Work out the finished part from the listing and answer in its coordinate system (mm). Face numbers are marked on the shaded views. A direction names the side the tool comes from. Coordinates: 2 decimals unless noted, no trailing zeros. Write each loop counter-clockwise with the first axis right and the second up, starting at its lowest first coordinate (ties: lowest second). Pieces come first, ordered by that corner, then holes. Notation, with made-up numbers: (-4.75, 19.25) - (54.25, 19.25) arc R15 ccw to (54.25, 36.25) - close; hole circle Ø3 at (79, 42). An arc over 180 degrees is marked (long way). Use a Markdown table: item, result. Add a question column.
(1) For a pull along Z with two mould halves and no side action, classify the marked faces 1, 2, 3 and 4 as released by +Z, released by -Z, zero draft, split by the parting line, or undercut.
(2) The part is cut by section A-A, the plane z = -13.5. Give the vertices of the cut face in (x, y).
(3) Find the intervals of material crossed by line 1 (Y direction, x = -0.2, z = -13.5); line 2 (Z direction, x = 2.25, y = -1); line 3 (Z direction, x = 0.25, y = -6), in increasing order. Write a range as from..to.
(4) The part is cut by section D-D, the plane z = -9. Give the vertices of the cut face in (x, y).
(5) Given pin 1 Ø1.8 at (x, y) = (-5, 1.5) entering from -Z; pin 2 Ø2 at (x, y) = (7, -7.5) entering from -Z; pin 3 Ø8 at (x, z) = (2, -9) entering from +Y, each flat-ended and moving along its own axis, determine where each tip first touches the part or whether it passes through.
(6) The part is cut by section B-B, the plane x = 0. Give the vertices of the cut face in (y, z).
(7) A tool of negligible diameter and unlimited length cuts with its end or side. For the marked faces 5, 6, 7 and 8, from which of +Z, -Z, +X, -X, +Y, -Y can it reach the whole face along a straight path? Write none if from no direction.
(8) The part is cut by section C-C, the plane y = 0. Give the vertices of the cut face in (x, z), then the cut area to 3 significant figures.
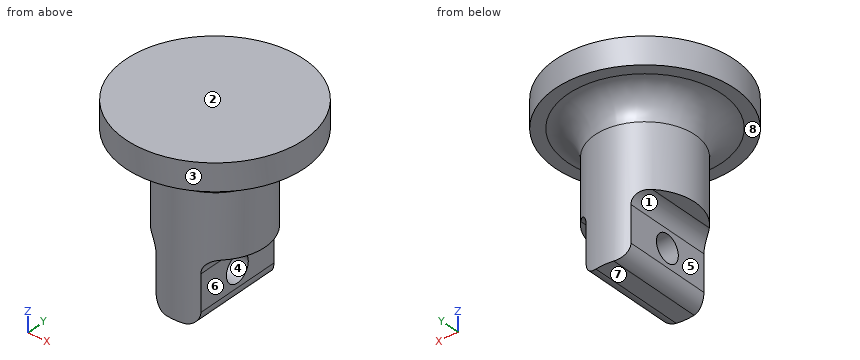
from build123d import *
from OCP.BRepFilletAPI import BRepFilletAPI_MakeFillet

# Parameters (mm, degrees)
SKETCH1_R           = 10
BOSS_EXTRUDE1_DEPTH = 3
SKETCH2_R           = 5.6
BOSS_EXTRUDE2_DEPTH = 17
CUT_EXTRUDE1_DEPTH  = 7
CUT_EXTRUDE2_REACH  = 25.351
SKETCH4_R           = 1.5
FILLET1_R1          = 3
FILLET1_R2          = 1.5


with BuildPart() as part:
    # Sketch1 → Boss-Extrude1 (new body)
    with BuildSketch(Plane.XY):
        Circle(SKETCH1_R)
    extrude(amount=BOSS_EXTRUDE1_DEPTH)

    # Sketch2 → Boss-Extrude2 (add)
    with BuildSketch(Plane(origin=(0, 0, 0), x_dir=(-1, 0, 0), z_dir=(0, 0, -1))):
        with Locations(Location((0, 0, 0), (0, 0, 180))):
            Circle(SKETCH2_R)
    extrude(amount=BOSS_EXTRUDE2_DEPTH)

    # Sketch3 → Cut-Extrude1 (cut)
    with BuildSketch(Plane(origin=(0, 0, -17), x_dir=(-1, 0, 0), z_dir=(0, 0, -1))):
        with BuildLine():
            Line((2.5, 0), (2.5, 6.663171691))
            ThreePointArc((2.5, 6.663171691), (8.066213365, -0.537352556), (2.5, -7.737876802))
            Line((2.5, -7.737876802), (2.5, 0))
        make_face()
        with BuildLine():
            Line((-2.5, 0), (-2.5, 6.663171691))
            ThreePointArc((-2.5, 6.663171691), (-7.668145551, -0.537352556), (-2.5, -7.737876802))
            Line((-2.5, -7.737876802), (-2.5, 0))
        make_face()
    extrude(amount=-CUT_EXTRUDE1_DEPTH, mode=Mode.SUBTRACT)

    # Sketch4 → Cut-Extrude2 (cut, up to next)
    with BuildSketch(Plane(origin=(2.5, 0, 0), x_dir=(0, 0, -1), z_dir=(1, 0, 0)), mode=Mode.PRIVATE) as cut_extrude2_sk1:
        with Locations((13.5, 0)):
            Circle(SKETCH4_R)
    cut_extrude2_tool1 = extrude(cut_extrude2_sk1.sketch, amount=-CUT_EXTRUDE2_REACH, mode=Mode.PRIVATE) & part.part
    add(cut_extrude2_tool1.solids().sort_by_distance((2.5, 0, -13.5))[0], mode=Mode.SUBTRACT)

    # Fillet1: one fillet with a radius per group of edges: ONE call of the kernel's fillet builder (fillet() takes one radius for all edges)
    fillet1_edges_1 = [part.edges().sort_by_distance(p)[0] for p in [
        (-5.6, 0, 0),
    ]]
    fillet1_edges_2 = [part.edges().sort_by_distance(p)[0] for p in [
        (2.5, 0, -10),
        (-2.5, 0, -10),
        (2.5, 0, -17),
        (-2.5, 0, -17),
    ]]
    fillet1 = BRepFilletAPI_MakeFillet(part.part.solid().wrapped)
    for e in fillet1_edges_1:
        fillet1.Add(FILLET1_R1, e.wrapped)
    for e in fillet1_edges_2:
        fillet1.Add(FILLET1_R2, e.wrapped)
    add(Compound.cast(fillet1.Shape()), mode=Mode.REPLACE)


solid = part.part
Model answer:
| question | item | result |
|---|---|---|
| 1 | face 1 | released by -Z |
| 1 | face 2 | released by +Z |
| 1 | face 3 | zero draft |
| 1 | face 4 | undercut |
| 2 | outline | (-2.5, -5.01) arc R5.6 ccw to (2.5, -5.01) - (2.5, -1.5) - (-2.5, -1.5) - close; (-2.5, 1.5) - (2.5, 1.5) - (2.5, 5.01) arc R5.6 ccw to (-2.5, 5.01) - close |
| 3 | line 1 | -5.6..-1.5, 1.5..5.6 |
| 3 | line 2 | -16.33..-14.62, -12.38..3 |
| 3 | line 3 | -1.49..3 |
| 4 | outline | circle Ø11.2 at (0, 0) |
| 5 | pin 1 | z = -10 |
| 5 | pin 2 | z = 0 |
| 5 | pin 3 | y = 5.6 |
| 6 | outline | (-10, 0) - (-8.6, 0) arc R3 cw to (-5.6, -3) - (-5.6, -17) - (5.6, -17) - (5.6, -3) arc R3 cw to (8.6, 0) - (10, 0) - (10, 3) - (-10, 3) - close; hole circle Ø3 at (0, -13.5) |
| 7 | face 5 | -Z, -X, +Y, -Y |
| 7 | face 6 | -Z, +X, +Y, -Y |
| 7 | face 7 | -Z, +X, -X, +Y, -Y |
| 7 | face 8 | -Z |
| 8 | outline | (-10, 0) - (-8.6, 0) arc R3 cw to (-5.6, -3) - (-5.6, -10) - (-4, -10) arc R1.5 cw to (-2.5, -11.5) - (-2.5, -12) - (2.5, -12) - (2.5, -11.5) arc R1.5 cw to (4, -10) - (5.6, -10) - (5.6, -3) arc R3 cw to (8.6, 0) - (10, 0) - (10, 3) - (-10, 3) - close; (-2.5, -15.5) arc R1.5 ccw to (-1, -17) - (1, -17) arc R1.5 ccw to (2.5, -15.5) - (2.5, -15) - (-2.5, -15) - close |
| 8 | area | 196 mm^2 |
